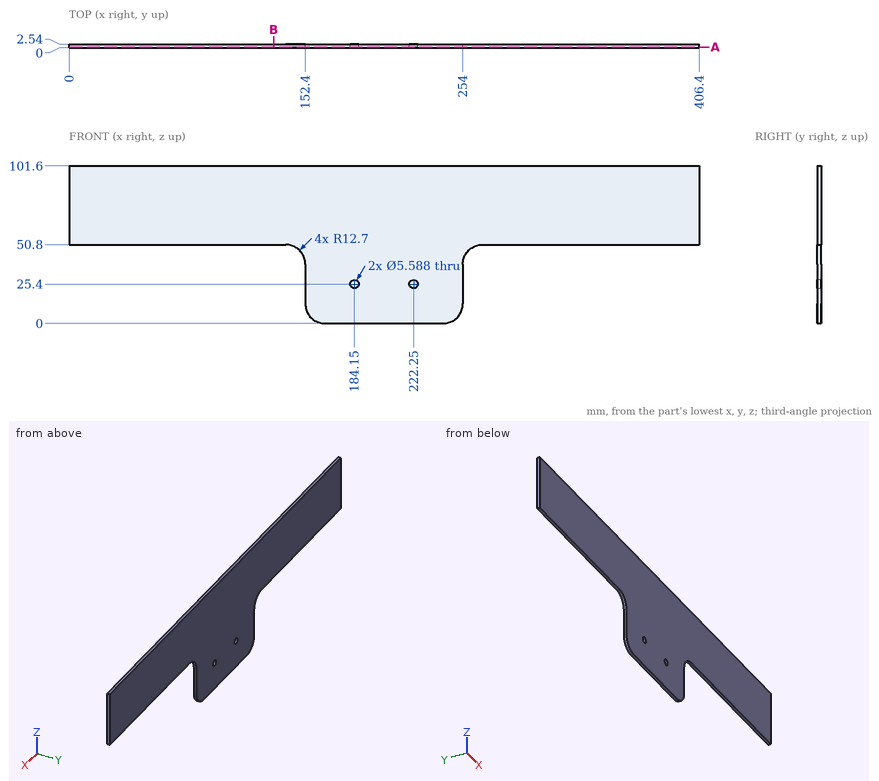
Part print with two shaded views. Sizes in mm from the minimum x, y, z corner. Round coordinates to 2 decimals unless told otherwise and drop trailing zeros. Order: outer loops, then holes, each group sorted by start corner. A loop starts at its lowest first (then second) coordinate and runs counter-clockwise, first axis right, second up. Notation, with made-up numbers: M 56,-16.75 L 92,-16.75 A21 ccw 92,0.25 Z; hole C 30.5,13.25 d6. An arc over 180 degrees is marked long. Use CSV: the item, a comma, the result in double quotes.
Item 1: Saw through at B-B (x = 132). List the corners of the cut face in (y, z).
Worked answers:
outline,"M 0,50.8 L 2.54,50.8 L 2.54,101.6 L 0,101.6 Z"
Item 2: Pin check, flat tips, straight feed: pin 1 (0.8 mm diameter, centred on y = 1.5, z = 25.5, fed in from +X); pin 2 (1.5 mm diameter, centred on x = 68, z = 62.5, fed in from -Y); pin 3 (1 mm diameter, centred on x = 102, y = 1, fed in from -Z). Stop position of each tip, or through.
Worked answers:
pin 1,"x = 254"
pin 2,"y = 0"
pin 3,"z = 50.8"
Item 3: Probe probe 1 along X at (y, z) = (1.1, 25.4); probe 2 along X at (y, z) = (0.8, 35.5); probe 3 along Z at (x, y) = (324, 0.95). List the from-to ranges inside material, lowest first.
Worked answers:
probe 1,"152.4 to 181.36, 186.94 to 219.46, 225.04 to 254"
probe 2,"152.4 to 254"
probe 3,"50.8 to 101.6"
Item 4: Saw through at A-A (y = 0.45). List the corners of the cut face in (x, z).
Worked answers:
outline,"M 0,50.8 L 139.7,50.8 A12.7 cw 152.4,38.1 L 152.4,12.7 A12.7 ccw 165.1,0 L 241.3,0 A12.7 ccw 254,12.7 L 254,38.1 A12.7 cw 266.7,50.8 L 406.4,50.8 L 406.4,101.6 L 0,101.6 Z; hole C 184.15,25.4 d5.59; hole C 222.25,25.4 d5.59"
